Build history of the part. All positions in model axes, mm. A direction names the side the tool comes from. Round coordinates to 2 decimals unless told otherwise and drop trailing zeros. Write each loop counter-clockwise with the first axis right and the second up, starting at its lowest first coordinate (ties: lowest second). Pieces come first, ordered by that corner, then holes. Notation, with made-up numbers: (-38.75, -24) -> (-31.75, -24) arc R19 cw to (-31.75, 4) -> close; hole circle Ø5 at (-7.5, -14.75). An arc over 180 degrees is marked (long way). One line per question, with ' | ' between items.
from build123d import *

# Parameters (mm, degrees)
F0_W         = 67.5
F0_H         = 20
F1_DEPTH     = 1
F2_W         = 71
F2_H         = 27
F3_DEPTH     = 1
F4_W         = 67.5
F4_H         = 20
F5_DEPTH     = 1
F6_R         = 0.99999
F7_R         = 1
F8_W         = 2
F8_H         = 15
F9_DEPTH     = 4
F10_T1_DEPTH = 26.4948974279
F11_SIZE     = 0.3


# Not quite as in the source:
# - a fillet or chamfer that OpenCascade refuses, or shapes differently, is made with other operations: its cross-section is extruded or revolved along the edge and cut away or added
# - a fillet or chamfer is up to 0.001 mm smaller than in the source, because OpenCascade refuses the exact size


with BuildPart() as f1:
    # F0 (on Top) → F1 (new body)
    with BuildSketch(Plane.XY):
        with Locations((-4.0991377383, -20.9536040443)):
            Rectangle(F0_W, F0_H)
    extrude(amount=F1_DEPTH)

    # F2 (on face) → F3 (join)
    with BuildSketch(Plane.XY.offset(1)):
        with Locations((-5.8491377383, -20.9536040443)):
            Rectangle(F2_W, F2_H)
    extrude(amount=F3_DEPTH)

    # F4 (on face) → F5 (join)
    with BuildSketch(Plane.XY.offset(2)):
        with Locations((-4.0991377383, -20.9536040443)):
            Rectangle(F4_W, F4_H)
    extrude(amount=F5_DEPTH)

    # F6 (radius 1 in the source; OpenCascade refuses exactly that, so slightly less here)
    f6_edges = [f1.edges().sort_by_distance(p)[0] for p in [
        (29.650862, -9.203604, 1),
        (29.650862, -32.703604, 1),
    ]]
    fillet(f6_edges, radius=F6_R)

    # F7
    f7_edges = [f1.edges().sort_by_distance(p)[0] for p in [
        (29.650862, -20.953604, 0),
    ]]
    fillet(f7_edges, radius=F7_R)

    # F8 (on face) → F9 (join)
    with BuildSketch(Plane(origin=(0, 0, 0), x_dir=(1, 0, 0), z_dir=(0, 0, -1))):
        with Locations((14.6508622617, 20.9536040443)):
            Rectangle(F8_W, F8_H)
    extrude(amount=F9_DEPTH)

    # F10: fillet of radius 5 on 2 edges, made by hand

    # F10_s2 → F10_t1 (cut)
    with BuildSketch(Plane.YZ.offset(1.4034135477)):
        with BuildLine():
            ThreePointArc((-28.4536040443, 0), (-26.7169022189, -2.8729833462), (-23.5546245587, -4))
            Line((-23.5546245587, -4), (-28.4536040443, -4))
            Line((-28.4536040443, -4), (-28.4536040443, 0))
        make_face()
        with BuildLine():
            ThreePointArc((-13.4536040443, 0), (-15.1903058697, -2.8729833462), (-18.3525835299, -4))
            Line((-18.3525835299, -4), (-13.4536040443, -4))
            Line((-13.4536040443, -4), (-13.4536040443, 0))
        make_face()
    extrude(amount=F10_T1_DEPTH, mode=Mode.SUBTRACT)

    # F11
    f11_edges = [f1.edges().sort_by_distance(p)[0] for p in [
        (-41.349138, -20.953604, 2),
        (-41.349138, -20.953604, 1),
    ]]
    chamfer(f11_edges, length=F11_SIZE)


solid = f1.part
(1) Slice it at B-B (x = -17.5). Write the cut outline in (y, z).
Calculated:
outline: (-34.45, 1) -> (-30.95, 1) -> (-30.95, 0) -> (-10.95, 0) -> (-10.95, 1) -> (-7.45, 1) -> (-7.45, 2) -> (-10.95, 2) -> (-10.95, 3) -> (-30.95, 3) -> (-30.95, 2) -> (-34.45, 2) -> close
(2) Wall check: line 1 (Z direction, x = -13.5, y = -29); line 2 (Y direction, x = -37, z = 2.25); line 3 (X direction, y = -26, z = -0.75). Give the ranges that are in metal, low to high. Write a range as from..to.
Calculated:
line 1: 0..3 | line 2: -30.95..-10.95 | line 3: 13.65..15.65
(3) 3-axis set-ups, long thin cutter, end or side, ignore diameter. For faces 1 (the flat face through (15.651, -21, -2)), 2 (the flat face through (13.651, -21, -2)), 3 (the cylindrical face through (14.637, -26.754, -2.842)): which of +Z, -Z, +X, -X, +Y, -Y reach the whole face in a straight line?
Calculated:
face 1: -Z, +X, +Y, -Y | face 2: -Z, -X, +Y, -Y | face 3: -Z, +X, -X, -Y
(4) Drop flat-ended pins along their axis: pin 1 (6 mm diameter, centred on x = 20, y = -30.5, fed in from -Z); pin 2 (1.1 mm diameter, centred on x = -19, z = 2.5, fed in from +Y); pin 3 (1.1 mm diameter, centred on y = -19, z = 0.5, fed in from -X); pin 4 (0.5 mm diameter, centred on x = -12.5, z = 2.5, fed in from -Y). Give the stop position or say it passes through.
Calculated:
pin 1: z = 0 | pin 2: y = -7.45 | pin 3: x = -41.1 | pin 4: y = -30.95
(5) Slice it at D-D (z = -3). Write the cut outline in (x, y).
Calculated:
outline: (13.65, -26.55) -> (15.65, -26.55) -> (15.65, -15.35) -> (13.65, -15.35) -> close
(6) Slice it at A-A (y = -21). Write the cut outline in (x, z).
Calculated:
outline: (-41.35, 1.3) -> (-41.05, 1) -> (-37.85, 1) -> (-37.85, 0) -> (13.65, 0) -> (13.65, -4) -> (15.65, -4) -> (15.65, 0) -> (28.65, 0) arc R1 ccw to (29.65, 1) -> (29.65, 3) -> (-37.85, 3) -> (-37.85, 2) -> (-41.05, 2) -> (-41.35, 1.7) -> close
